from build123d import *

# Parameters (mm, degrees)
SKETCH2_R           = 3.25
SKETCH2_R_2         = 2.15
BOSS_EXTRUDE1_DEPTH = 5


with BuildPart() as part:
    # Sketch2 → Boss-Extrude1 (new body)
    with BuildSketch(Plane.XY):
        with BuildLine():
            ThreePointArc((58.247868643, 87.353936938), (70.038600193, 111.62640422), (43.670645638, 105.890117005))
            add(Edge.make_bspline(
                [(43.670645638, 105.890117005), (15.172778081, 91.437929288), (-14.968147584, 82.320982869), (-46.752131357, 78.539277748)],
                knots=[0, 0, 0, 0, 1, 1, 1, 1], degree=3, weights=[1, 1, 1, 1]))
            add(Edge.make_bspline(
                [(-46.752131357, 78.539277748), (-78.53611513, 82.320982869), (-108.677040795, 91.437929288), (-137.174908352, 105.890117005)],
                knots=[0, 0, 0, 0, 1, 1, 1, 1], degree=3, weights=[1, 1, 1, 1]))
            ThreePointArc((-137.174908352, 105.890117005), (-163.542862908, 111.62640422), (-151.752131357, 87.353936938))
            add(Edge.make_bspline(
                [(-151.752131357, 87.353936938), (-137.251152171, 67.836975358), (-128.318856179, 46.170308692), (-124.955243383, 22.353936938)],
                knots=[0, 0, 0, 0, 1, 1, 1, 1], degree=3, weights=[1, 1, 1, 1]))
            add(Edge.make_bspline(
                [(-124.955243383, 22.353936938), (-128.318856179, -1.462434816), (-137.251152171, -23.129101482), (-151.752131357, -42.646063062)],
                knots=[0, 0, 0, 0, 1, 1, 1, 1], degree=3, weights=[1, 1, 1, 1]))
            ThreePointArc((-151.752131357, -42.646063062), (-163.542862908, -66.918530344), (-137.174908352, -61.182243129))
            add(Edge.make_bspline(
                [(-137.174908352, -61.182243129), (-108.677040795, -46.730055412), (-78.53611513, -37.613108993), (-46.752131357, -33.831403872)],
                knots=[0, 0, 0, 0, 1, 1, 1, 1], degree=3, weights=[1, 1, 1, 1]))
            add(Edge.make_bspline(
                [(-46.752131357, -33.831403872), (-14.968147584, -37.613108993), (15.172778081, -46.730055412), (43.670645638, -61.182243129)],
                knots=[0, 0, 0, 0, 1, 1, 1, 1], degree=3, weights=[1, 1, 1, 1]))
            ThreePointArc((43.670645638, -61.182243129), (70.038600194, -66.918530344), (58.247868643, -42.646063062))
            add(Edge.make_bspline(
                [(58.247868643, -42.646063062), (43.746889456, -23.129101482), (34.814593465, -1.462434816), (31.450980669, 22.353936938)],
                knots=[0, 0, 0, 0, 1, 1, 1, 1], degree=3, weights=[1, 1, 1, 1]))
            add(Edge.make_bspline(
                [(31.450980669, 22.353936938), (34.814593465, 46.170308692), (43.746889456, 67.836975358), (58.247868643, 87.353936938)],
                knots=[0, 0, 0, 0, 1, 1, 1, 1], degree=3, weights=[1, 1, 1, 1]))
        make_face()
        with Locations((-151.752131357, 102.353936938)):
            Circle(SKETCH2_R, mode=Mode.SUBTRACT)
        with Locations((58.247868643, -57.646063062)):
            Circle(SKETCH2_R, mode=Mode.SUBTRACT)
        with Locations((58.247868643, 102.353936938)):
            Circle(SKETCH2_R, mode=Mode.SUBTRACT)
        with Locations((-1.752131357, 22.353936938)):
            Circle(SKETCH2_R_2, mode=Mode.SUBTRACT)
        with Locations((-91.752131357, 22.353936938)):
            Circle(SKETCH2_R_2, mode=Mode.SUBTRACT)
        with Locations((-151.752131357, -57.646063062)):
            Circle(SKETCH2_R, mode=Mode.SUBTRACT)
    extrude(amount=BOSS_EXTRUDE1_DEPTH)


solid = part.part
Input: part model. Units: mm. Frame: model coordinates. Coordinates: 2 decimals unless noted, no trailing zeros. Write item = value, one per line. Start each with the question number.
(1) Line query: line 1 along Y through (x, z) = (-153, 0.35); line 2 along Y through (x, z) = (41.5, 2.6); line 3 along Y through (x, z) = (44.5, 3.5). Output: solid intervals per line, ascending. Write a range as [from, to].
(2) Pull-direction query (Y, two-part tool) for faces 1 (the flat face through (-48, 24, 5)), 2 (the cylindrical face through (70.323, 111.253, 2.465)); classes: released by +Y, released by -Y, zero draft, split by the parting line, or undercut.
(3) Section A-A on z = 3.95. Give the number of separate pieces and of enclosed holes in the cut face, and give its area (3 significant figures).
(4) First-contact query: P1, Ø6, axis at x = 58.25, y = 102.35, coming from the +Z side; P2, Ø1.5, axis at y = 62, z = 3, coming from the -X side; P3, Ø1, axis at y = 52.5, z = 3.5, coming from the -X side; P4, Ø2, axis at y = 89.5, z = 2, coming from the +X side. Flat tips, straight axial feed; report the tip coordinate or a pass-through.
Result set:
q1.line_1 = [-72.59, -60.65], [-54.65, -42.7], [87.41, 99.35], [105.35, 117.3]
q1.line_2 = [-60.09, -13.72], [58.43, 104.8]
q1.line_3 = [-63.65, -20.22], [64.93, 108.35]
q2.face_1 = zero draft
q2.face_2 = undercut
q3.separate_pieces = 1
q3.enclosed_holes = 6
q3.area = 26,500 mm²
q4.P1 = through
q4.P2 = -136.95
q4.P3 = -132.8
q4.P4 = 67.44
